Check sheet for the modelled part. Datum: model origin and axes. Units: mm. Face numbers are marked on the shaded views. A direction names the side the tool comes from. Round coordinates to 2 decimals unless told otherwise and drop trailing zeros. Loops run counter-clockwise (first coordinate to the right, second up) from the corner with the lowest first, then second, coordinate; pieces in that order, holes last. Notation, with made-up numbers: (3, -37.5) -> (38, -37.5) arc R20 cw to (38, -16.5) -> close; hole circle Ø11 at (-34, 4). An arc over 180 degrees is marked (long way). Use one line per item in the form item = value. Start each with the question number.
(1) Sectioned sample at B-B (z = 26.5). Record the cut outline in (x, y), and give its area (3 significant figures).
(2) Sectioned sample at C-C (z = 50). Record the cut outline in (x, y), and give its area (3 significant figures).
(3) Set-up check for the marked faces 1 and 2: record each of +Z, -Z, +X, -X, +Y, -Y from which the full face is reachable in a straight line by a thin tool's end or side.
(4) Material ranges on probe 1 along X at (y, z) = (2, 51); probe 2 along Y at (x, z) = (-1.5, 34); probe 3 along X at (y, z) = (-0.25, 18), recorded low to high. Write a range as [from, to].
(5) Go/stop test with flat-tipped pins: pin 1 (2 mm diameter, centred on x = 5.5, z = 31.5, fed in from +Y); pin 2 (4 mm diameter, centred on x = -6.5, z = 62.5, fed in from -Y); pin 3 (8 mm diameter, centred on y = -6, z = 15.5, fed in from +X). Record where each tip stops, or that it passes through.
(6) Sectioned sample at D-D (z = 60). Record the cut outline in (x, y).
(7) Sectioned sample at A-A (x = 0). Record the cut outline in (y, z), and give its area (3 significant figures).
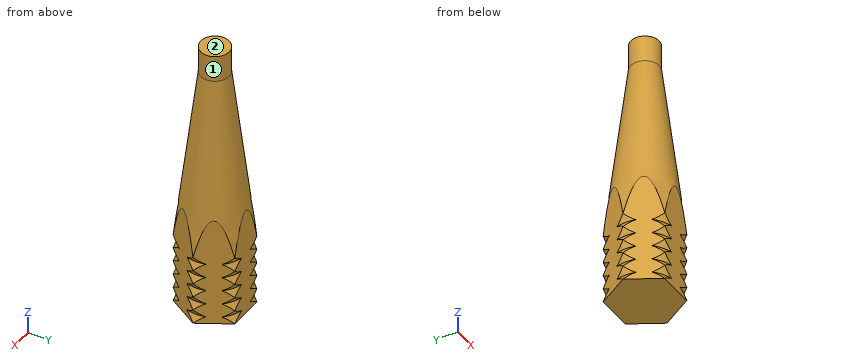
from build123d import *

# Parameters (mm, degrees)
F1_DEPTH = 20
F4_DEPTH = 25
F7_DEPTH = 1


with BuildPart() as f1:
    # F0 (on Top) → F1 (new body)
    with BuildSketch(Plane.XY):
        Polygon((10, 0), (5, 8.6602540378), (-5, 8.6602540378), (-10, 0), (-5, -8.6602540378), (5, -8.6602540378), align=None)
    extrude(amount=F1_DEPTH)

    # F2 (on Right) → F3 (revolve)
    with BuildSketch(Plane.YZ):
        Polygon((-4, 76.5), (-4, 70), (-10, 20), (0, 20), (0, 70), (0, 76.5), align=None)
    revolve(axis=Axis((0, 0, 45), (0, 0, 1)))

    # F4 (cut): faces of the model
    f4_faces = [f1.faces().sort_by_distance(p)[0] for p in [
        (-7.9668740123, 4.5996768556, 20),
        (0, 9.1993537112, 20),
        (-7.9668740123, -4.5996768556, 20),
        (0, -9.1993537112, 20),
        (7.9668740123, -4.5996768556, 20),
        (7.9668740123, 4.5996768556, 20),
    ]]
    extrude(f4_faces, amount=-F4_DEPTH, mode=Mode.SUBTRACT)

    # F5 (on Front) → F6 (revolve, cut)
    with BuildSketch(Plane.XZ):
        Polygon((-8.8642183308, 18), (-10, 20), (-10, 16), align=None)
        Polygon((-8.8642183308, 2), (-10, 4), (-10, 0), align=None)
        Polygon((-8.8642183308, 6), (-10, 8), (-10, 4), align=None)
        Polygon((-8.8642183308, 10), (-10, 12), (-10, 8), align=None)
        Polygon((-8.8642183308, 14), (-10, 16), (-10, 12), align=None)
    revolve(axis=Axis((0, 0, 5.5472087115), (0, 0, -1)), mode=Mode.SUBTRACT)

    # F7 (add): a face of the model
    f7_faces = [f1.faces().sort_by_distance(p)[0] for p in [
        (0, 0, 76.5),
    ]]
    extrude(f7_faces, amount=F7_DEPTH)


solid = f1.part
Checks:
q1.outline = (-9.08, -1.59) -> (-5.92, -7.07) arc R9.22 ccw to (-3.16, -8.66) -> (3.16, -8.66) arc R9.22 ccw to (5.92, -7.07) -> (9.08, -1.59) arc R9.22 ccw to (9.08, 1.59) -> (5.92, 7.07) arc R9.22 ccw to (3.16, 8.66) -> (-3.16, 8.66) arc R9.22 ccw to (-5.92, 7.07) -> (-9.08, 1.59) arc R9.22 ccw to start
q1.area = 253 mm2
q2.outline = circle Ø12.8 at (0, 0)
q2.area = 129 mm2
q3.face_1 = +Z
q3.face_2 = +Z, +X, -X, +Y, -Y
q4.probe_1 = [-5.95, 5.95]
q4.probe_2 = [-8.18, 8.18]
q4.probe_3 = [-8.86, 8.86]
q5.pin_1 = 7.37
q5.pin_2 = -1.98
q5.pin_3 = 8.85
q6.outline = circle Ø10.4 at (0, 0)
q7.outline = (-8.66, 0) -> (8.66, 0) -> (8.66, 31.16) -> (4, 70) -> (4, 77.5) -> (-4, 77.5) -> (-4, 70) -> (-8.66, 31.16) -> close
q7.area = 1,090 mm2
